Geometry check sheet. Reference: the model listing, model coordinates, mm. A direction names the side the tool comes from. Coordinates: 2 decimals unless noted, no trailing zeros. Loops run counter-clockwise (first coordinate to the right, second up) from the corner with the lowest first, then second, coordinate; pieces in that order, holes last.
from build123d import *

# Parameters (mm, degrees)
F0_W     = 5.842
F0_H     = 12.7
F0_R     = 3.175
F2_DEPTH = 3.175
F3_R     = 1.524
F4_DEPTH = 7.62


with BuildPart() as f1:
    # F0 (on Front) → F1 (revolve)
    with BuildSketch(Plane.XZ):
        Polygon((5.842, 12.7), (5.842, 0), (66.294, 0), (66.294, 12.7), (56.134, 12.7), (56.134, 10.16), (10.16, 10.16), (10.16, 12.7), align=None)
    revolve(axis=Axis((33.147, 0, 0), (-1, 0, 0)))

    # F0 (on Front) → F2 (join, symmetric)
    with BuildSketch(Plane.XZ):
        with Locations((2.921, 6.35)):
            Rectangle(F0_W, F0_H)
        with BuildLine():
            Line((-0.9398, 0), (0, 0))
            Line((0, 0), (0, 12.7))
            Line((0, 12.7), (5.842, 12.7))
            Line((5.842, 12.7), (5.842, 15.24))
            Line((5.842, 15.24), (-0.508, 15.24))
            Line((-0.508, 15.24), (-10.8806298187, 3.8475430269))
            ThreePointArc((-10.8806298187, 3.8475430269), (-4.5919612295, 5.3297205562), (-0.9398, 0))
        make_face()
        with BuildLine():
            ThreePointArc((-8.1826630726, -5.5069827884), (-3.1957909266, -4.5493385486), (-0.9398, 0))
            ThreePointArc((-0.9398, 0), (-4.5919612295, 5.3297205562), (-10.8806298187, 3.8475430269))
            ThreePointArc((-10.8806298187, 3.8475430269), (-12.1459778134, -1.5837270034), (-8.1826630726, -5.5069827884))
        make_face()
        with Locations((-6.6548, 0)):
            Circle(F0_R, mode=Mode.SUBTRACT)
        with BuildLine():
            Line((5.842, 0), (0, 0))
            Line((0, 0), (-0.9398, 0))
            ThreePointArc((-0.9398, 0), (-3.1957909266, -4.5493385486), (-8.1826630726, -5.5069827884))
            Line((-8.1826630726, -5.5069827884), (5.842, -9.398))
            Line((5.842, -9.398), (5.842, 0))
        make_face()
    extrude(amount=F2_DEPTH, both=True)

    # F3 (on face) → F4 (join)
    with BuildSketch(Plane.YZ.offset(66.294)):
        with BuildLine():
            Line((-4.9956931261, 11.6761744673), (-5.0798671661, 0.0367365628))
            ThreePointArc((-5.0798671661, 0.0367365628), (-0.0197170397, 5.0799617359), (5.0794289447, 0.0761682073))
            Line((5.0794289447, 0.0761682073), (5.0794289447, 11.6399914775))
            ThreePointArc((5.0794289447, 11.6399914775), (0.0456094729, 12.6999181012), (-4.9956931261, 11.6761744673))
        make_face()
        with BuildLine():
            ThreePointArc((5.0794289447, 0.0761682073), (-0.0197170397, 5.0799617359), (-5.0798671661, 0.0367365628))
            ThreePointArc((-5.0798671661, 0.0367365628), (-0.0564528103, -5.0796863171), (5.0794289447, -0.0761682073))
            Line((5.0794289447, -0.0761682073), (5.0794289447, 0.0761682073))
        make_face()
        Circle(F3_R, mode=Mode.SUBTRACT)
        with BuildLine():
            Line((-4.9710357562, 15.0857521221), (-4.9956931261, 11.6761744673))
            ThreePointArc((-4.9956931261, 11.6761744673), (0.0456094729, 12.6999181012), (5.0794289447, 11.6399914775))
            Line((5.0794289447, 11.6399914775), (5.0794289447, 15.1638317927))
            Line((5.0794289447, 15.1638317927), (-4.9710357562, 15.0857521221))
        make_face()
    extrude(amount=F4_DEPTH)


solid = f1.part
(1) Draft check along Y on faces 1 (the flat face through (66.294, 0, 0)), 2 (the flat face through (70, 5.079, 7)), 3 (the cylindrical face through (70.051, -0.168, -5.077)), 4 (the cylindrical face through (70.05, -0.2, 1.51)). Enter one of: +Y half, -Y half, draft (parallel to the pull), parting line (faces both ways), or undercut.
Findings:
face 1: undercut
face 2: +Y half
face 3: parting line
face 4: undercut
(2) Sectioned sample at C-C on x = 49. Record the cut outline in (y, z), and give its area (3 significant figures).
Findings:
outline: circle Ø20.32 at (0, 0)
area: 324 mm2
(3) Access from +Z, -Z, +X, -X, +Y, -Y to the whole of each face (thin tool, end or side, straight path). Record for faces 5 (the flat face through (-1, 3.175, 3)), 6 (the flat face through (-1, -3.175, 3)), 7 (the cylindrical face through (-12.168, -0.044, -1.505)), 8 (the flat face through (10.16, 9, 6)).
Findings:
face 5: +Z, -Z, -X, +Y
face 6: +Z, -Z, -X, -Y
face 7: -X, +Y, -Y
face 8: none
(4) Gauge pin test, flat ends, axial feed: pin 1 Ø12.5 at (y, z) = (2, -2.5) entering from -X; pin 2 Ø5 at (x, z) = (47.5, -7) entering from -Y; pin 3 Ø4 at (x, z) = (45.5, 1) entering from +Y; pin 4 Ø2 at (y, z) = (-7.5, -5.5) entering from -X. Record the tip position at first contact, or that the pin passes through.
Findings:
pin 1: stops at x = -12.37
pin 2: stops at y = -9.11
pin 3: stops at y = 10.16
pin 4: stops at x = 5.84
(5) Sectioned sample at B-B on y = -6.5. Record the cut outline in (x, z), and give its area (3 significant figures).
Findings:
outline: (5.84, -10.91) - (10.16, -10.91) - (10.16, -7.81) - (56.13, -7.81) - (56.13, -10.91) - (66.29, -10.91) - (66.29, 10.91) - (56.13, 10.91) - (56.13, 7.81) - (10.16, 7.81) - (10.16, 10.91) - (5.84, 10.91) - close
area: 1,030 mm2
(6) Sectioned sample at A-A on z = 9. Record the cut outline in (x, y) (3 decimals), and give its area (3 significant figures).
Findings:
outline: (-6.189, -3.175) - (5.842, -3.175) - (5.842, -8.96) - (10.16, -8.96) - (10.16, -4.714) - (56.134, -4.714) - (56.134, -8.96) - (66.294, -8.96) - (66.294, -5.015) - (73.914, -5.015) - (73.914, 5.079) - (66.294, 5.079) - (66.294, 8.96) - (56.134, 8.96) - (56.134, 4.714) - (10.16, 4.714) - (10.16, 8.96) - (5.842, 8.96) - (5.842, 3.175) - (-6.189, 3.175) - close
area: 846 mm2
(7) Scan lines: L1, parallel to X at y = 1.25, z = -10.75; L2, parallel to X at y = 0, z = 14.25; L3, parallel to Z at x = 68.75, y = 0. Record each from-to range of solid material in increasing order.
Findings:
L1: x = 5.84 to 10.16, 56.13 to 66.29
L2: x = -1.41 to 5.84, 66.29 to 73.91
L3: z = -5.08 to -1.52, 1.52 to 15.12
